Read the model definition and answer for the solid it produces. Units are mm, in the model's axes. A direction names the side the tool comes from. Round coordinates to 2 decimals unless told otherwise and drop trailing zeros. Write each loop counter-clockwise with the first axis right and the second up, starting at its lowest first coordinate (ties: lowest second). Pieces come first, ordered by that corner, then holes. Notation, with made-up numbers: (9.5, 50.25) -> (37.5, 50.25) arc R21 ccw to (37.5, 62.25) -> close; hole circle Ø9 at (15.25, 65.25). An arc over 180 degrees is marked (long way). Return JSON: item names as keys, results as strings. Group by question number.
(1) A cutting plane is placed at A-A on z = 2.3. State how many separate pieces and enclosed holes the cut face has, then the cut area to 3 significant figures.
(2) A cutting plane is placed at B-B on x = 18.5. Give the vertices of the cut face in (y, z), then the cut area to 3 significant figures.
(3) The mould has two halves that part along X. Classify faces 1 (the flat face through (0, -18.9, 3)), 2 (the cylindrical face through (-33.74, 21.2, 0.81)), 3 (the cylindrical face through (33.7, 21.24, 0.81)), 4 (the flat face through (31.4, 0, 3)): released by +X, released by -X, zero draft, split by the parting line, or undercut.
(4) For faces 5 (the flat face through (33, 0, 3)), 6 (the flat face through (0, 0, 1.6)), 7 (the flat face through (0, 20.5, 3)), 8 (the flat face through (-33, 0, 3)), determine the directions among +Z, -Z, +X, -X, +Y, -Y from which every point of the face is accessible in a straight line to the end or side of a thin tool.
(5) Given pin 1 (2 mm diameter, centred on x = -11.5, z = 3.5, fed in from -Y); pin 2 (1.4 mm diameter, centred on y = 6, z = 3, fed in from -X); pin 3 (12 mm diameter, centred on x = 25, y = -4, fed in from +Z), each flat-ended and moving along its own axis, determine where each tip first touches the part or whether it passes through.
(6) A cutting plane is placed at D-D on y = 18. Give the vertices of the cut face in (x, z), then the cut area to 3 significant figures.
(7) A cutting plane is placed at C-C on y = -1.5. Give the vertices of the cut face in (x, z).
(8) Straight lines are drawn through the part: line 1 (Y direction, x = 24, z = 3.75); line 2 (X direction, y = -12, z = 2); line 3 (Z direction, x = 23.5, y = -14). For each, find the intervals that lie inside material, in ascending order.
```python
from build123d import *

# Parameters (mm, degrees)
F0_W     = 69.2
F0_H     = 44.2
F1_DEPTH = 1.6
F2_W     = 59.2
F2_H     = 1.6
F2_W_2   = 1.6
F2_H_2   = 34.2
F3_DEPTH = 2.8
F4_R     = 3
F5_R     = 0.79999


# Not quite as in the source:
# - a fillet or chamfer is up to 0.001 mm smaller than in the source, because OpenCascade refuses the exact size


with BuildPart() as f1:
    # F0 (on Top) → F1 (new body)
    with BuildSketch(Plane.XY):
        Rectangle(F0_W, F0_H)
    extrude(amount=F1_DEPTH)

    # F2 (on face) → F3 (join)
    with BuildSketch(Plane.XY.offset(1.6)):
        with Locations((0, -19.7)):
            Rectangle(F2_W, F2_H)
        with Locations((-32.2, 0)):
            Rectangle(F2_W_2, F2_H_2)
        with Locations((32.2, 0)):
            Rectangle(F2_W_2, F2_H_2)
        with Locations((0, 19.7)):
            Rectangle(F2_W, F2_H)
    extrude(amount=F3_DEPTH)

    # F4
    f4_edges = [f1.edges().sort_by_distance(p)[0] for p in [
        (34.6, -22.1, 0.8),
        (34.6, 22.1, 0.8),
        (-34.6, -22.1, 0.8),
        (-34.6, 22.1, 0.8),
    ]]
    fillet(f4_edges, radius=F4_R)

    # F5 (radius 0.8 in the source; OpenCascade refuses exactly that, so slightly less here)
    f5_edges = [f1.edges().sort_by_distance(p)[0] for p in [
        (29.6, -20.5, 3),
        (29.6, -18.9, 3),
        (33, -17.1, 3),
        (31.4, -17.1, 3),
        (29.6, 18.9, 3),
        (29.6, 20.5, 3),
        (-33, -17.1, 3),
        (-31.4, 17.1, 3),
        (-31.4, -17.1, 3),
        (-29.6, 18.9, 3),
        (31.4, 17.1, 3),
        (33, 17.1, 3),
        (-33, 17.1, 3),
        (-29.6, -18.9, 3),
        (-29.6, 20.5, 3),
        (-29.6, -20.5, 3),
    ]]
    fillet(f5_edges, radius=F5_R)


solid = f1.part
```
Checks:
{
 "1": {"separate pieces": "4", "enclosed holes": "0", "area": "297 mm^2"},
 "2": {"outline": "(-22.1, 0) -> (22.1, 0) -> (22.1, 1.6) -> (20.5, 1.6) -> (20.5, 4.4) -> (18.9, 4.4) -> (18.9, 1.6) -> (-18.9, 1.6) -> (-18.9, 4.4) -> (-20.5, 4.4) -> (-20.5, 1.6) -> (-22.1, 1.6) -> close", "area": "79.7 mm^2"},
 "3": {"face 1": "zero draft", "face 2": "released by -X", "face 3": "released by +X", "face 4": "undercut"},
 "4": {"face 5": "+Z, +X, +Y, -Y", "face 6": "+Z", "face 7": "+Z, +X, -X, +Y", "face 8": "+Z, -X, +Y, -Y"},
 "5": {"pin 1": "stops at y = -20.5", "pin 2": "stops at x = -33", "pin 3": "stops at z = 1.6"},
 "6": {"outline": "(-34.6, 0) -> (34.6, 0) -> (34.6, 1.6) -> (-34.6, 1.6) -> close", "area": "111 mm^2"},
 "7": {"outline": "(-34.6, 0) -> (34.6, 0) -> (34.6, 1.6) -> (33, 1.6) -> (33, 4.4) -> (31.4, 4.4) -> (31.4, 1.6) -> (-31.4, 1.6) -> (-31.4, 4.4) -> (-33, 4.4) -> (-33, 1.6) -> (-34.6, 1.6) -> close"},
 "8": {"line 1": "y = -20.5 to -18.9, 18.9 to 20.5", "line 2": "x = -33 to -31.4, 31.4 to 33", "line 3": "z = 0 to 1.6"}
}
